from build123d import *

# Parameters (mm, degrees)
SKETCH1_R          = 6.25
SKETCH1_R_2        = 1.575
BASE_FLANGE1_DEPTH = 3
L_EK1_SCALE        = 2


# Sheet-metal steps are written as plain solids
with BuildPart() as part:
    # Sketch1 → Base-Flange1 (new body)
    with BuildSketch(Plane(origin=(0, 0, 0), x_dir=(1, 0, 0), z_dir=(0, 1, 0))):
        with BuildLine():
            Line((19.609421573, -14.059417906), (10.862109445, -29.480175346))
            ThreePointArc((10.862109445, -29.480175346), (9.762567662, -30.59234701), (8.252687872, -31))
            Line((8.252687872, -31), (-8.352599575, -31))
            ThreePointArc((-8.352599575, -31), (-9.796606082, -30.629609326), (-10.884048227, -29.609896806))
            Line((-10.884048227, -29.609896806), (-20.742852548, -14.107625594))
            ThreePointArc((-20.742852548, -14.107625594), (-21.091885276, -13.336076582), (-21.211403896, -12.497728788))
            Line((-21.211403896, -12.497728788), (-21.211403896, 14.839305313))
            ThreePointArc((-21.211403896, 14.839305313), (-21.044943633, 15.824725306), (-20.564035521, 16.700789784))
            Line((-20.564035521, 16.700789784), (-10.150833328, 29.861484472))
            ThreePointArc((-10.150833328, 29.861484472), (-9.105019706, 30.700412322), (-7.798201703, 31))
            Line((-7.798201703, 31), (7.702138241, 31))
            ThreePointArc((7.702138241, 31), (9.077698333, 30.666052219), (10.147014932, 29.738556288))
            Line((10.147014932, 29.738556288), (19.444876691, 16.663267527))
            ThreePointArc((19.444876691, 16.663267527), (19.857851472, 15.837226972), (20, 14.924711239))
            Line((20, 14.924711239), (20, -12.57924256))
            ThreePointArc((20, -12.57924256), (19.900712388, -13.344662472), (19.609421573, -14.059417906))
        make_face()
        with Locations(Location((7.5, -13.4, 0), (0, 0, 270))):
            Circle(SKETCH1_R, mode=Mode.SUBTRACT)
        with Locations(Location((6, -27, 0), (0, 0, 270))):
            Circle(SKETCH1_R_2, mode=Mode.SUBTRACT)
        with Locations(Location((-6, -27, 0), (0, 0, 270))):
            Circle(SKETCH1_R_2, mode=Mode.SUBTRACT)
        with Locations(Location((5.25, 27.940782939, 0), (0, 0, 270))):
            Circle(SKETCH1_R_2, mode=Mode.SUBTRACT)
        with Locations(Location((-5.25, 27.940782939, 0), (0, 0, 270))):
            Circle(SKETCH1_R_2, mode=Mode.SUBTRACT)
        with Locations(Location((13.5, 7.05, 0), (0, 0, 270))):
            Circle(SKETCH1_R_2, mode=Mode.SUBTRACT)
        with Locations(Location((-13.5, 7.05, 0), (0, 0, 270))):
            Circle(SKETCH1_R_2, mode=Mode.SUBTRACT)
        with BuildLine():
            Line((-13.281403896, 0), (-13.281403896, 1.54698652))
            ThreePointArc((-13.281403896, 1.54698652), (-10.122330587, 2.700024029), (-8.222660082, 5.475))
            Line((-8.222660082, 5.475), (8.230334451, 5.475))
            ThreePointArc((8.230334451, 5.475), (10.061414817, 2.757432943), (13.113110627, 1.563624456))
            ThreePointArc((13.113110627, 1.563624456), (14.07117407, -0.953003234), (11.655254401, -2.142386538))
            ThreePointArc((11.655254401, -2.142386538), (0.639353267, -3.554619032), (-4.5, -13.4))
            ThreePointArc((-4.5, -13.4), (-8.890701948, -17.790701948), (-13.281403896, -13.4))
            Line((-13.281403896, -13.4), (-13.281403896, 0))
        make_face(mode=Mode.SUBTRACT)
        with BuildLine():
            Line((-8.222660082, 8.625), (8.230334451, 8.625))
            ThreePointArc((8.230334451, 8.625), (9.780248168, 11.101351171), (12.37962963, 12.434679214))
            ThreePointArc((12.37962963, 12.434679214), (0.003755557, 20.549999478), (-12.376631792, 12.441566144))
            ThreePointArc((-12.376631792, 12.441566144), (-9.773901449, 11.105506282), (-8.222660082, 8.625))
        make_face(mode=Mode.SUBTRACT)
    extrude(amount=BASE_FLANGE1_DEPTH)


with BuildPart() as part_1:
    # Ölçek1: scaled about (-0.5271359, 1.5, 0.12162837)
    add(part.part.scale(L_EK1_SCALE).moved(Location((0.5271359, -1.5, -0.12162837))))


solid = part_1.part
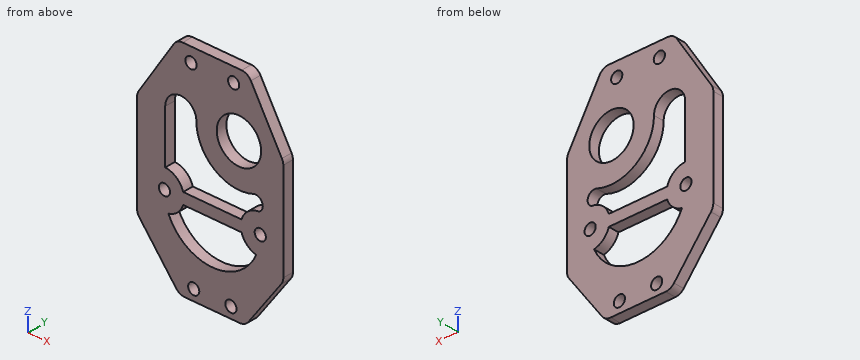
Source: CAD feature listing. Evaluate the final solid. Frame: model axes, mm. Coordinates: 2 decimals unless noted, no trailing zeros. Loops run counter-clockwise (first coordinate to the right, second up) from the corner with the lowest first, then second, coordinate; pieces in that order, holes last. Notation, with made-up numbers: M 36.25,5 L 66.25,5 A15 cw 66.25,17 Z; hole C 7.5,-21 d5. An arc over 180 degrees is marked long. Answer in a Markdown table with one row per item.
Q1. Section B-B on z = 22. Return the cut outline in (x, y).
Answers below:
| item | result |
|---|---|
| outline | M -41.9,-1.5 L -26.04,-1.5 L -26.04,4.5 L -41.9,4.5 Z; M -8.01,-1.5 L 3.94,-1.5 L 3.94,4.5 L -8.01,4.5 Z; M 27.12,-1.5 L 40.53,-1.5 L 40.53,4.5 L 27.12,4.5 Z |
Q2. First-contact query: pin 1 (3 mm diameter, centred on x = -20.5, y = 3.5, fed in from -Z); pin 2 (2 mm diameter, centred on y = 2, z = -47, fed in from -X); pin 3 (5 mm diameter, centred on x = 11.03, z = -56, fed in from +Y). Flat tips, straight axial feed; report the tip coordinate or a pass-through.
Answers below:
| item | result |
|---|---|
| pin 1 | stops at z = -60.65 |
| pin 2 | stops at x = -30.73 |
| pin 3 | passes through |
Q3. Section D-D on x = -36. Return the cut outline in (y, z).
Answers below:
| item | result |
|---|---|
| outline | M -1.5,-39.34 L 4.5,-39.34 L 4.5,35.89 L -1.5,35.89 Z |
Q4. Section C-C on x = 6. Return the cut outline in (y, z), plus the area to 3 significant figures.
Answers below:
| item | result |
|---|---|
| outline | M -1.5,-62.12 L 4.5,-62.12 L 4.5,-40.66 L -1.5,-40.66 Z; M -1.5,-17.37 L 4.5,-17.37 L 4.5,-11.07 L -1.5,-11.07 Z; M -1.5,4.65 L 4.5,4.65 L 4.5,18.59 L -1.5,18.59 Z; M -1.5,34.77 L 4.5,34.77 L 4.5,61.88 L -1.5,61.88 Z |
| area | 413 mm^2 |
Q5. Section A-A on y = 3.35. State how many separate pieces and enclosed holes the cut face has, plus the area to 3 significant figures.
Answers below:
| item | result |
|---|---|
| separate pieces | 1 |
| enclosed holes | 9 |
| area | 5,930 mm^2 |
Q6. Ray query, probe 1 along Z at (x, y) = (13.5, 1.65); probe 2 along Z at (x, y) = (19, 0.65); probe 3 along Z at (x, y) = (-22.5, 2.75). Return the intervals inside material, ascending. Write a range as from..to.
Answers below:
| item | result |
|---|---|
| probe 1 | z = -62.12..-57.95, -54.05..-37.9, -17.37..-11.07, 2.76..14.34, 39.01..50.88, 56.87..61.88 |
| probe 2 | z = -61.28..-33.91, -21.17..-7.27, 2.93..14.67, 38.69..61.55 |
| probe 3 | z = -56.4..-28.32, -24.49..-3.95, 33.72..57.12 |
